from build123d import *

# Parameters (mm, degrees)
F0_R     = 5
F0_R_2   = 2.5
F0_R_3   = 1
F1_DEPTH = 1.5
F2_DEPTH = 3
F3_R     = 5
F4_DEPTH = 5


with BuildPart() as f1:
    # F0 (on Top) → F1 (new body)
    with BuildSketch(Plane.XY):
        Circle(F0_R)
        Circle(F0_R_2, mode=Mode.SUBTRACT)
        Circle(F0_R_2)
        Circle(F0_R_3, mode=Mode.SUBTRACT)
    extrude(amount=F1_DEPTH)

    # F0 (on Top) → F2 (join)
    with BuildSketch(Plane.XY):
        Circle(F0_R)
        Circle(F0_R_2, mode=Mode.SUBTRACT)
    extrude(amount=-F2_DEPTH)

    # F3 (on face) → F4 (join)
    with BuildSketch(Plane.XY.offset(1.5)):
        Circle(F3_R)
        Polygon((-3.046816, 0.894564), (-0.748693, 3.085902), (2.298123, 2.191338), (3.046816, -0.894564), (0.748693, -3.085902), (-2.298123, -2.191338), align=None, mode=Mode.SUBTRACT)
    extrude(amount=F4_DEPTH)


solid = f1.part
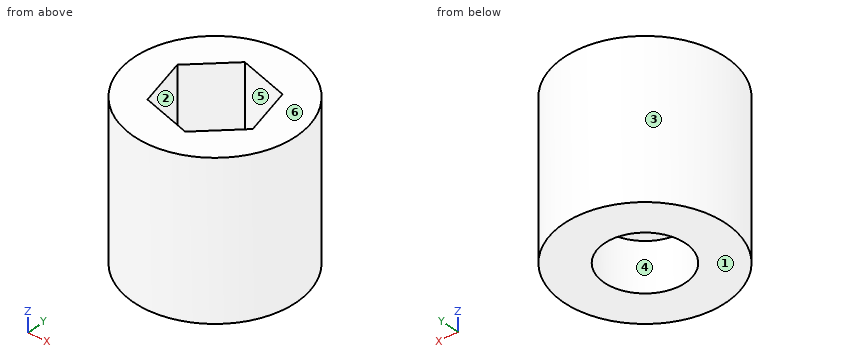
Design review of the part built by this model. Coordinates are the model's own, in mm. Face numbers are marked on the shaded views. A direction names the side the tool comes from. Round coordinates to 2 decimals unless told otherwise and drop trailing zeros. Write each loop counter-clockwise with the first axis right and the second up, starting at its lowest first coordinate (ties: lowest second). Pieces come first, ordered by that corner, then holes. Notation, with made-up numbers: M 57,-36 L 111,-36 A34 cw 111,0 Z; hole C -11,79.25 d5. An arc over 180 degrees is marked long. One line per item, written item: value. Start each with the question number.
1. Take a section at B-B on x = 0. State the section outline as (y, z) points.
2. Take a section at C-C on y = 0.25. State the section outline as (x, z) points.
3. Take a section at D-D on y = -2.75. State the section outline as (x, z) points, then the cut area to 3 significant figures.
4. Clearance check with flat-ended pins moving along their axes: P1, Ø1.5, axis at x = 0, y = 1, coming from the +Z side; P2, Ø1.5, axis at y = -2, z = -1.5, coming from the -X side. State where each tip first meets the part, or that it passes through.
5. Draft analysis for pull direction Y (two halves, no side actions). For the marked faces 1, 2 and 3, state which applies: pulls with the +Y half, pulls with the -Y half, needs draft (parallel to the pull), parting line crosses it, or undercut.
6. To check wall thickness, follow probe 1 along Y at (x, z) = (0, 0.5); probe 2 along Y at (x, z) = (0, -2.3); probe 3 along Z at (x, y) = (-0.5, -1.25). State the ranges of each line that lie inside material, in increasing order. Write a range as from..to.
7. Take a section at A-A on z = 5. State the section outline as (x, y) points, then the cut area to 3 significant figures.
8. For the marked faces 4, 5 and 6, list the 3-axis set-ups (+Z, -Z, +X, -X, +Y, -Y) from which the entire face can be reached by the end or side of a thin tool; tool diameter is ignored.
Computed:
1. outline: M -5,-3 L -2.5,-3 L -2.5,0 L -1,0 L -1,1.5 L -2.87,1.5 L -2.87,6.5 L -5,6.5 Z; M 1,0 L 2.5,0 L 2.5,-3 L 5,-3 L 5,6.5 L 2.87,6.5 L 2.87,1.5 L 1,1.5 Z
2. outline: M -4.99,-3 L -2.49,-3 L -2.49,0 L -0.97,0 L -0.97,1.5 L -2.89,1.5 L -2.89,6.5 L -4.99,6.5 Z; M 0.97,0 L 2.49,0 L 2.49,-3 L 4.99,-3 L 4.99,6.5 L 2.77,6.5 L 2.77,1.5 L 0.97,1.5 Z
3. outline: M -4.18,-3 L 4.18,-3 L 4.18,6.5 L 1.1,6.5 L 1.1,1.5 L -0.4,1.5 L -0.4,6.5 L -4.18,6.5 Z
3. area: 71.9 mm²
4. P1: stops at z = 1.5
4. P2: stops at x = -4.84
5. face 1: needs draft
5. face 2: undercut
5. face 3: parting line crosses it
6. probe 1: y = -5..-1, 1..5
6. probe 2: y = -5..-2.5, 2.5..5
6. probe 3: z = 0..1.5
7. outline: C 0,0 d10; hole M -3.05,0.89 L -2.3,-2.19 L 0.75,-3.09 L 3.05,-0.89 L 2.3,2.19 L -0.75,3.09 Z
7. area: 52.3 mm²
8. face 4: -Z
8. face 5: +Z
8. face 6: +Z, +X, -X, +Y, -Y
